from build123d import *

# Parameters (mm, degrees)
SKETCH1_R           = 18.5
SKETCH1_R_2         = 17.5
SKETCH1_R_3         = 4.5
SKETCH1_R_4         = 3.5
BOSS_EXTRUDE1_DEPTH = 1
SKETCH2_R           = 18.5
SKETCH2_R_2         = 17.5
BOSS_EXTRUDE2_DEPTH = 15
BOSS_EXTRUDE3_DEPTH = 1


with BuildPart() as part:
    # Sketch1 → Boss-Extrude1 (new body)
    with BuildSketch(Plane(origin=(0, 0, 0), x_dir=(1, 0, 0), z_dir=(0, 1, 0))):
        with Locations(Location((0, 0, 0), (0, 0, 270))):
            Circle(SKETCH1_R)
        Circle(SKETCH1_R_2, mode=Mode.SUBTRACT)
        Circle(SKETCH1_R_3)
        with Locations(Location((0, 0, 0), (0, 0, 270))):
            Circle(SKETCH1_R_4, mode=Mode.SUBTRACT)
        with BuildLine():
            Line((0, 17.5), (0, 4.5))
            ThreePointArc((0, 4.5), (3.181980515, 3.181980515), (4.5, 0))
            ThreePointArc((4.5, 0), (3.181980515, -3.181980515), (0, -4.5))
            Line((0, -4.5), (0, -17.5))
            ThreePointArc((0, -17.5), (12.374368671, -12.374368671), (17.5, 0))
            ThreePointArc((17.5, 0), (12.374368671, 12.374368671), (0, 17.5))
        make_face()
    extrude(amount=BOSS_EXTRUDE1_DEPTH)

    # Sketch2 → Boss-Extrude2 (add)
    with BuildSketch(Plane(origin=(0, 1, 0), x_dir=(1, 0, 0), z_dir=(0, 1, 0))):
        with Locations(Location((0, 0, 0), (0, 0, 270))):
            Circle(SKETCH2_R)
        with Locations(Location((0, 0, 0), (0, 0, 270))):
            Circle(SKETCH2_R_2, mode=Mode.SUBTRACT)
    extrude(amount=BOSS_EXTRUDE2_DEPTH)

    # Sketch3 → Boss-Extrude3 (add)
    with BuildSketch(Plane(origin=(0, 16, 0), x_dir=(1, 0, 0), z_dir=(0, 1, 0))):
        with BuildLine():
            Line((0, 18.5), (0, -18.5))
            ThreePointArc((0, -18.5), (-18.5, 0), (0, 18.5))
        make_face()
    extrude(amount=BOSS_EXTRUDE3_DEPTH)


solid = part.part
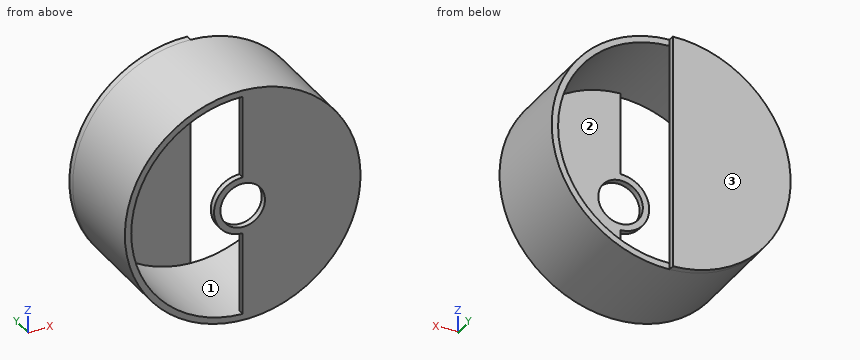
Could you check a few things on this model? Use its own coordinates, in mm. Face numbers are marked on the shaded views. Coordinates: 2 decimals unless noted, no trailing zeros. Loops run counter-clockwise (first coordinate to the right, second up) from the corner with the lowest first, then second, coordinate; pieces in that order, holes last.
1. Imagine slicing it at C-C (x = 1.5). Please give me the cut outline in (y, z).
2. Imagine slicing it at A-A (z = 0). Please give me the cut outline in (x, y).
3. Imagine slicing it at B-B (x = 8.5). Please give me the cut outline in (y, z), and give its area (3 significant figures).
4. I need wall thicknesses on L1, parallel to X at y = 0.2, z = 0; L2, parallel to X at y = 12.5, z = 0. Which ranges of each line are inside material? Lowest first, please.
5. Imagine slicing it at D-D (y = 13.25). Please give me the cut outline in (x, z).
6. For P1, Ø0.8, axis at y = 16.5, z = 7, coming from the +X side; P2, Ø5.5, axis at x = 12.5, z = -2.5, coming from the +Y side; P3, Ø8, axis at x = -5, y = 4.5, coming from the -Z side, each with a flat end and sliding along its axis, tell me the tip position at first contact or that it passes through.
7. We'd pull the mould along Z, two halves only. Please class the marked faces 1, 2 and 3: released by +Z, released by -Z, zero draft, split by the parting line, or undercut.
Computed values:
1. outline: (0, -18.44) - (16, -18.44) - (16, -17.44) - (1, -17.44) - (1, -3.16) - (0, -3.16) - close; (0, 3.16) - (1, 3.16) - (1, 17.44) - (16, 17.44) - (16, 18.44) - (0, 18.44) - close
2. outline: (-18.5, 0) - (-17.5, 0) - (-17.5, 16) - (0, 16) - (0, 17) - (-18.5, 17) - close; (-4.5, 0) - (-3.5, 0) - (-3.5, 1) - (-4.5, 1) - close; (3.5, 0) - (18.5, 0) - (18.5, 16) - (17.5, 16) - (17.5, 1) - (3.5, 1) - close
3. outline: (0, -16.43) - (16, -16.43) - (16, -15.3) - (1, -15.3) - (1, 15.3) - (16, 15.3) - (16, 16.43) - (0, 16.43) - close
3. area: 66.9 mm2
4. L1: x = -18.5 to -17.5, -4.5 to -3.5, 3.5 to 18.5
4. L2: x = -18.5 to -17.5, 17.5 to 18.5
5. outline: circle Ø37 at (0, 0); hole circle Ø35 at (0, 0)
6. P1: stops at x = 0
6. P2: stops at y = 1
6. P3: stops at z = -18.47
7. face 1: undercut
7. face 2: undercut
7. face 3: zero draft
